Autodesk Inventor part; units mm, degrees
ref_plane "YZ Plane" through (0, 0, 0) normal (1, 0, 0) x (0, 1, 0)
ref_plane "XZ Plane" through (0, 0, 0) normal (0, 1, 0) x (-1, 0, 0)
ref_plane "XY Plane" through (0, 0, 0) normal (0, 0, 1) x (1, 0, 0)
sketch "Sketch1" plane through (0, 0, 0) normal (0, 1, 0) x (-1, 0, 0)
  line L0 (125, 30) -> (-125, 30)
  line L1 (-125, 30) -> (-125, -30)
  line L2 (-125, -30) -> (125, -30)
  line L3 (125, -30) -> (125, 30)
  line L4 (125, 30) -> (-125, -30) construction
  line L5 (-125, 30) -> (125, -30) construction
  point P0 (0, 0)
  dimension "d0" = 250
  dimension "d1" = 60
extrude "Extrusion1" add sketch "Sketch1" along normal mid plane 3
sketch "Sketch2" plane through (0, -1.5, 0) normal (0, -1, 0) x (1, 0, 0)
  line L0 (125, -30) -> (125, 30)
  line L1 (125, 30) -> (-125, 30)
  line L2 (-125, 30) -> (-125, -30)
  point P0 (0, 0)
  point P1 (113.5, 15)
  point P2 (113.5, -15)
  point P3 (-113.5, 15)
  point P4 (-113.5, -15)
  dimension "d9" = 11.5
  dimension "d10" = 15
  dimension "d11" = 30
  dimension "d12" = 11.5
hole "Hole1" at (113.5, -1.5, 15) at (113.5, -1.5, -15) at (-113.5, -1.5, 15) at (-113.5, -1.5, -15) direction (0, 1, 0) diameter 4.4587 depth 12.8 tip angle 118
sketch "Sketch3" plane through (0, 1.5, 0) normal (0, 1, 0) x (1, 0, 0)
  line L0 (125, -23.3203) -> (125, -25.9184)
  line L1 (125, 30) -> (-125, 30)
  line L2 (-125, 30) -> (-125, -30)
  line L3 (125, 30) -> (-125, 30)
  line L4 (-125, 30) -> (-125, 25)
  line L5 (-125, 25) -> (125, 25)
  line L6 (125, 25) -> (125, 30)
  point P0 (0, 0)
  point P1 (125, 28.5858)
  dimension "d20" = 5
extrude "Extrusion2" cut sketch "Sketch3" against normal blind 3
properties part number "2309HCMUTE-CDT23_TAM-GA" material "PMMA Plastic"
CAD build for the part. Positions are in the model's coordinates, mm. Coordinates: 2 decimals unless noted, no trailing zeros. Write each loop counter-clockwise with the first axis right and the second up, starting at its lowest first coordinate (ties: lowest second). Pieces come first, ordered by that corner, then holes. Notation, with made-up numbers: (-8.75, -10) -> (18.25, -10) arc R16 cw to (18.25, 19) -> close; hole circle Ø3 at (-21.5, 2.5). An arc over 180 degrees is marked (long way). Use CSV: the item, a comma, the result in double quotes. Start each with the question number.
Item 1: Wall check: probe 1 along Z at (x, y) = (-113.5, 0.5); probe 2 along X at (y, z) = (0.65, -15); probe 3 along X at (y, z) = (0, -16.5). Give the ranges that are in metal, low to high.
Item 2: Two-plate mould, pull along X, no slides. Class faces 1 (the cylindrical face through (-111.324, 0.021, -14.517)), 2 (the flat face through (2, 1.5, 3)): +X half, -X half, draft (parallel to the pull), parting line (faces both ways), or undercut.
Item 3: Band-saw the part on B-B, the plane z = 15. Write the cut outline in (x, y), plus the area to 3 significant figures.
Item 4: Band-saw the part on A-A, the plane x = 113.5. Write the cut outline in (y, z).
Response values:
1,probe 1,"z = -25 to -17.23, -12.77 to 12.77, 17.23 to 30"
1,probe 2,"x = -125 to -115.73, -111.27 to 111.27, 115.73 to 125"
1,probe 3,"x = -125 to -115.15, -111.85 to 111.85, 115.15 to 125"
2,face 1,"undercut"
2,face 2,"draft"
3,outline,"(-125, -1.5) -> (-115.73, -1.5) -> (-115.73, 1.5) -> (-125, 1.5) -> close; (-111.27, -1.5) -> (111.27, -1.5) -> (111.27, 1.5) -> (-111.27, 1.5) -> close; (115.73, -1.5) -> (125, -1.5) -> (125, 1.5) -> (115.73, 1.5) -> close"
3,area,"723 mm2"
4,outline,"(-1.5, -25) -> (1.5, -25) -> (1.5, -17.23) -> (-1.5, -17.23) -> close; (-1.5, -12.77) -> (1.5, -12.77) -> (1.5, 12.77) -> (-1.5, 12.77) -> close; (-1.5, 17.23) -> (1.5, 17.23) -> (1.5, 30) -> (-1.5, 30) -> close"
